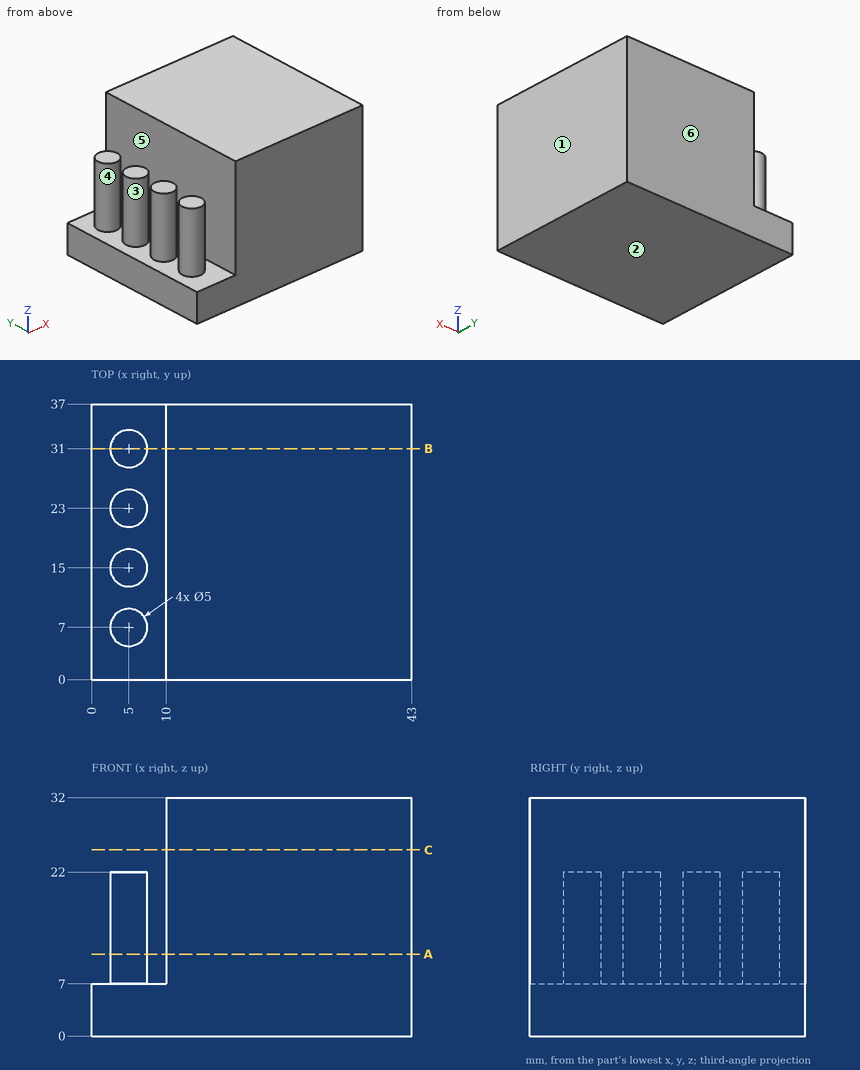
Job drawing, mm, ordinate dimensions from the low corner. One solid piece. A direction names the side the tool comes from. Coordinates: 2 decimals unless noted, no trailing zeros. Write each loop counter-clockwise with the first axis right and the second up, starting at its lowest first coordinate (ties: lowest second). Pieces come first, ordered by that corner, then holes. Notation, with made-up numbers: (74, 62.5) -> (103, 62.5) arc R33 cw to (103, 93.5) -> close; hole circle Ø3 at (67.5, 60). An arc over 180 degrees is marked (long way). Use CSV: the item, a comma, the result in double quotes. Start each with the question number.
Item 1: Drop flat-ended pins along their axis: P1, Ø1.5, axis at x = 5, y = 30.5, coming from the +Z side; P2, Ø3, axis at y = 33, z = 15.5, coming from the -X side; P3, Ø3, axis at x = 2.5, y = 10.5, coming from the +Z side. Give the stop position or say it passes through.
Item 2: Two-plate mould, pull along X, no slides. Class the marked faces 1, 2 and 3: +X half, -X half, draft (parallel to the pull), parting line (faces both ways), or undercut.
Item 3: Wall check: probe 1 along Z at (x, y) = (2.5, 27); probe 2 along X at (y, z) = (35, 18); probe 3 along Z at (x, y) = (5.5, 25). Give the ranges that are in metal, low to high.
Item 4: Band-saw the part on B-B, the plane y = 31. Write the cut outline in (x, z), plus the area to 3 significant figures.
Item 5: Band-saw the part on A-A, the plane z = 11. Write the cut outline in (x, y).
Item 6: Band-saw the part on C-C, the plane z = 25. Write the cut outline in (x, y).
Item 7: Tool access for the marked faces 4, 5 and 6: list every direction of +Z, -Z, +X, -X, +Y, -Y with a clear straight run to the whole face (end or side of a thin tool).
Response values:
1,P1,"stops at z = 22"
1,P2,"stops at x = 2.55"
1,P3,"stops at z = 7"
2,face 1,"+X half"
2,face 2,"draft"
2,face 3,"undercut"
3,probe 1,"z = 0 to 7"
3,probe 2,"x = 10 to 43"
3,probe 3,"z = 0 to 22"
4,outline,"(0, 0) -> (43, 0) -> (43, 32) -> (10, 32) -> (10, 7) -> (7.5, 7) -> (7.5, 22) -> (2.5, 22) -> (2.5, 7) -> (0, 7) -> close"
4,area,"1,200 mm2"
5,outline,"circle Ø5 at (5, 7); circle Ø5 at (5, 15); circle Ø5 at (5, 23); circle Ø5 at (5, 31); (10, 0) -> (43, 0) -> (43, 37) -> (10, 37) -> close"
6,outline,"(10, 0) -> (43, 0) -> (43, 37) -> (10, 37) -> close"
7,face 4,"+Z"
7,face 5,"+Z, +Y, -Y"
7,face 6,"+Z, -Z, +X, -X, +Y"
